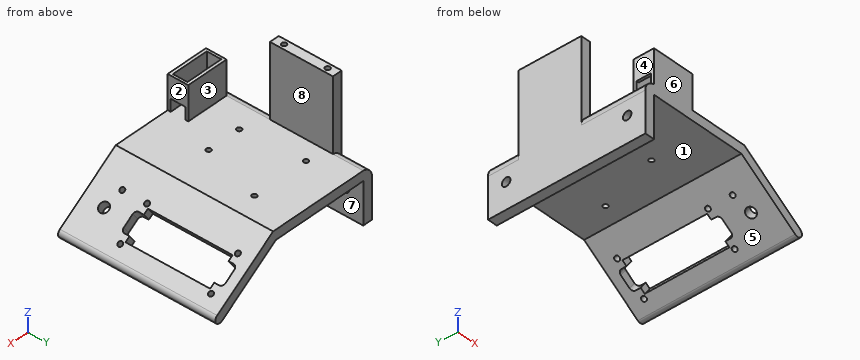
from build123d import *

# Parameters (mm, degrees)
F1_DEPTH       = 80
F1_DEPTH_BACK  = 50
F2_R           = 2
F3_DEPTH       = 25
F4_R           = 2
F5_DEPTH       = 25
F6_W           = 35
F6_H           = 17
F6_W_2         = 31
F6_H_2         = 12
F7_DEPTH       = 28
F8_W           = 6
F8_H           = 10
F9_DEPTH       = 43.001
F10_R          = 4
F10_R_2        = 2
F11_DEPTH      = 25
F12_R          = 3.5
F13_DEPTH      = 8
F14_W          = 8
F14_H          = 52
F15_DEPTH      = 60
F15_DEPTH_BACK = 25
F16_R          = 2
F17_DEPTH      = 25


with BuildPart() as f1:
    # F0 (on Front) → F1 (new body, two sides)
    with BuildSketch(Plane.XZ) as f1_sk:
        with BuildLine():
            Line((40, 34.4145861811), (89.1491226573, 0))
            ThreePointArc((89.1491226573, 0), (94.7200365799, 0.9823024318), (93.7377341481, 6.5532163543))
            Line((93.7377341481, 6.5532163543), (42.522390311, 42.4145861811))
            Line((42.522390311, 42.4145861811), (-40, 42.4145861811))
            ThreePointArc((-40, 42.4145861811), (-45.7082039325, 39.4703142711), (-48, 33.4703142711))
            Line((-48, 33.4703142711), (-48, 0))
            Line((-48, 0), (-40, 0))
            Line((-40, 0), (-40, 34.4145861811))
            Line((-40, 34.4145861811), (40, 34.4145861811))
        make_face()
    extrude(amount=F1_DEPTH)
    extrude(f1_sk.sketch, amount=-F1_DEPTH_BACK)

    # F2 (on face) → F3 (cut)
    with BuildSketch(Plane(origin=(33.9177749652, 0, 48.4396027096), x_dir=(0.8191520443, 0, -0.5735764364), z_dir=(0.5735764364, 0, 0.8191520443))):
        with BuildLine():
            Line((35.5266860713, 35), (35.5266860713, -35))
            Line((35.5266860713, -35), (40.0266860713, -35))
            Line((40.0266860713, -35), (40.0266860713, -39))
            ThreePointArc((40.0266860713, -39), (40.9053657278, -41.1213203436), (43.0266860713, -42))
            Line((43.0266860713, -42), (53.0266860713, -42))
            ThreePointArc((53.0266860713, -42), (55.1480064149, -41.1213203436), (56.0266860713, -39))
            Line((56.0266860713, -39), (56.0266860713, -35))
            Line((56.0266860713, -35), (60.5266860713, -35))
            Line((60.5266860713, -35), (60.5266860713, 35))
            Line((60.5266860713, 35), (56.0266860713, 35))
            Line((56.0266860713, 35), (40.0266860713, 35))
            Line((40.0266860713, 35), (35.5266860713, 35))
        make_face()
        with BuildLine():
            Line((40.0266860713, 35.0351855159), (40.0266860713, 35))
            Line((40.0266860713, 35), (56.0266860713, 35))
            Line((56.0266860713, 35), (56.0266860713, 39))
            ThreePointArc((56.0266860713, 39), (55.1480064149, 41.1213203436), (53.0266860713, 42))
            Line((53.0266860713, 42), (43.0266860713, 42))
            ThreePointArc((43.0266860713, 42), (40.9053657278, 41.1213203436), (40.0266860713, 39))
            Line((40.0266860713, 39), (40.0266860713, 35.0351855159))
        make_face()
        with Locations((33.0266860713, -37.5)):
            Circle(F2_R)
        with Locations((33.0266860713, 37.5)):
            Circle(F2_R)
        with Locations((63.0266860713, 37.5)):
            Circle(F2_R)
        with Locations((63.0266860713, -37.5)):
            Circle(F2_R)
    extrude(amount=-F3_DEPTH, mode=Mode.SUBTRACT)

    # F4 (on face) → F5 (cut)
    with BuildSketch(Plane.XY.offset(42.4145861811)):
        with Locations((8, -34.4999909401)):
            Circle(F4_R)
        with Locations((-20, -34.4999909401)):
            Circle(F4_R)
        with Locations((23.5, 17.4000090599)):
            Circle(F4_R)
        with Locations((-23.7, 17.4000090599)):
            Circle(F4_R)
    extrude(amount=-F5_DEPTH, mode=Mode.SUBTRACT)

    # F6 (on face) → F7 (join)
    with BuildSketch(Plane.XY.offset(42.4145861811)):
        with Locations((-22.5, -71.5)):
            Rectangle(F6_W, F6_H)
        with Locations((-22.5, -71.5)):
            Rectangle(F6_W_2, F6_H_2, mode=Mode.SUBTRACT)
    extrude(amount=F7_DEPTH)

    # F8 (on face) → F9 (cut, through all)
    with BuildSketch(Plane.YZ.offset(-5)):
        with Locations((-74.5, 47.4145861811)):
            Rectangle(F8_W, F8_H)
        with Locations((-68.5, 47.4145861811)):
            Rectangle(F8_W, F8_H)
    extrude(amount=-F9_DEPTH, mode=Mode.SUBTRACT)

    # F10 (on face) → F11 (cut)
    with BuildSketch(Plane(origin=(33.9177749652, 0, 48.4396027096), x_dir=(0.8191520443, 0, -0.5735764364), z_dir=(0.5735764364, 0, 0.8191520443))):
        with Locations((48.0266860713, -62)):
            Circle(F10_R)
        with Locations((33.0266860713, -58)):
            Circle(F10_R_2)
    extrude(amount=-F11_DEPTH, mode=Mode.SUBTRACT)

    # F12 (on face) → F13 (cut, through all)
    with BuildSketch(Plane(origin=(-48, 0, 0), x_dir=(0, -1, 0), z_dir=(-1, 0, 0))):
        with Locations((-35, 21.4703142711)):
            Circle(F12_R)
        with Locations((65, 21.4703142711)):
            Circle(F12_R)
    extrude(amount=-F13_DEPTH, mode=Mode.SUBTRACT)

    # F14 (on face) → F15 (join, two sides)
    with BuildSketch(Plane.XY.offset(42.4145861811)) as f15_sk:
        with Locations((-44, -1.0492918789)):
            Rectangle(F14_W, F14_H)
    extrude(amount=F15_DEPTH)
    extrude(f15_sk.sketch, amount=-F15_DEPTH_BACK)

    # F16 (on face) → F17 (cut)
    with BuildSketch(Plane.XY.offset(102.4145861811)):
        with Locations((-44, -19.0492918789)):
            Circle(F16_R)
        with Locations((-44, 16.9507081211)):
            Circle(F16_R)
    extrude(amount=-F17_DEPTH, mode=Mode.SUBTRACT)


solid = f1.part
Geometry: final body of the model. Coordinates: model frame, mm. Face numbers are marked on the shaded views. A direction names the side the tool comes from. Coordinates: 2 decimals unless noted, no trailing zeros. Order: outer loops, then holes, each group sorted by start corner. A loop starts at its lowest first (then second) coordinate and runs counter-clockwise, first axis right, second up.
1) Set-up query: the marked faces 1, 2, 3 and 4. Return all of +Z, -Z, +X, -X, +Y, -Y with unobstructed straight access to the full face (end or side cutting, diameter ignored); none if empty.
Result sheet:
face 1: -Z, +Y, -Y
face 2: +Z, +X, +Y, -Y
face 3: +Z, +X, -X, +Y
face 4: +Z, -X, -Y
2) Section C-C (y = -1). Return loops of the section in (x, z).
Result sheet:
outline: (-48, 0) - (-40, 0) - (-40, 34.41) - (40, 34.41) - (58.43, 21.51) - (63.02, 28.06) - (42.52, 42.41) - (-40, 42.41) - (-40, 102.41) - (-48, 102.41) - close; (78.91, 7.17) - (89.15, 0) arc R4 ccw to (93.74, 6.55) - (83.5, 13.72) - close
3) First-contact query: P1, Ø13.5, axis at y = -73, z = 58.5, coming from the +X side; P2, Ø6.5, axis at x = 23.5, y = 17.4, coming from the +Z side; P3, Ø6.5, axis at x = -46, z = 80.5, coming from the -Y side. Flat tips, straight axial feed; report the tip coordinate or a pass-through.
Result sheet:
P1: stops at x = -5
P2: stops at z = 42.41
P3: stops at y = -27.05
4) Ray query, probe 1 along Y at (x, z) = (-44, 91.25); probe 2 along Y at (x, z) = (-32, 59); probe 3 along X at (y, z) = (9, 87). Return the intervals inside material, ascending.
Result sheet:
probe 1: y = -27.05 to -21.05, -17.05 to 14.95, 18.95 to 24.95
probe 2: y = -80 to -77.5, -65.5 to -63
probe 3: x = -48 to -40
5) Section A-A (z = 46). Return loops of the section in (x, y), then the cut area to 3 significant figures.
Result sheet:
outline: (-48, -27.05) - (-40, -27.05) - (-40, 24.95) - (-48, 24.95) - close; (-40, -80) - (-5, -80) - (-5, -77.5) - (-40, -77.5) - close; (-40, -65.5) - (-5, -65.5) - (-5, -63) - (-40, -63) - close
area: 591 mm2
6) Draft query along X for the marked faces 5, 6, 7 and 8. Return one class per face: released by +X, released by -X, zero draft, split by the parting line, or undercut.
Result sheet:
face 5: undercut
face 6: zero draft
face 7: undercut
face 8: released by +X
7) Section D-D (x = -30). Return loops of the section in (y, z), then the cut area to 3 significant figures.
Result sheet:
outline: (-80, 34.41) - (50, 34.41) - (50, 42.41) - (-63, 42.41) - (-63, 70.41) - (-65.5, 70.41) - (-65.5, 42.41) - (-77.5, 42.41) - (-77.5, 70.41) - (-80, 70.41) - close
area: 1,180 mm2
8) Section B-B (x = 23.5). Return loops of the section in (y, z), then the cut area to 3 significant figures.
Result sheet:
outline: (-80, 34.41) - (15.4, 34.41) - (15.4, 42.41) - (-80, 42.41) - close; (19.4, 34.41) - (50, 34.41) - (50, 42.41) - (19.4, 42.41) - close
area: 1,010 mm2
